The drawing under review shows one solid part. Ordinate dimensions are in mm from its lowest x, y, z. Round coordinates to 2 decimals unless told otherwise and drop trailing zeros. Order: outer loops, then holes, each group sorted by start corner. A loop starts at its lowest first (then second) coordinate and runs counter-clockwise, first axis right, second up. Notation, with made-up numbers: M -18.75,32.5 L 28.25,32.5 A19 ccw 28.25,41.5 Z; hole C 22.25,85.5 d4. An arc over 180 degrees is marked long. Answer as a JSON object with one key per item and string values.
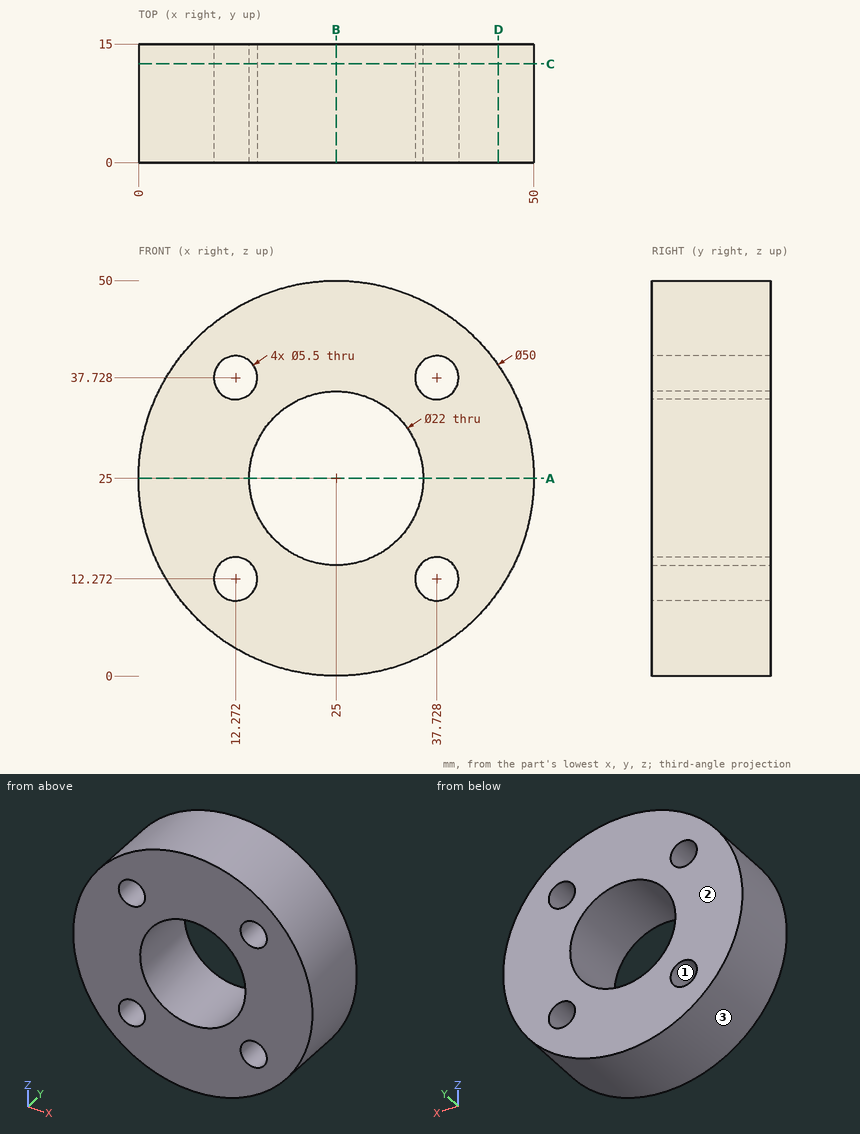
1) Add section D-D on x = 45.5. State the section outline as (y, z) points, and give its area (3 significant figures).
Geometry check:
{"outline": "M 0,10.69 L 15,10.69 L 15,39.31 L 0,39.31 Z", "area": "429 mm²"}
2) Insertion check: P1, Ø7, axis at x = 37.73, z = 12.27, coming from the -Y side; P2, Ø5, axis at x = 43.5, y = 12, coming from the -Z side; P3, Ø8, axis at x = 16.5, y = 13, coming from the -Z side; P4, Ø1, axis at x = 31, y = 12, coming from the +Z side. Each pin has a flat end and moves straight along its axis. Give the tip position at first contact, or say it passes through.
Geometry check:
{"P1": "stops at y = 0", "P2": "stops at z = 5.79", "P3": "stops at z = 0.41", "P4": "stops at z = 49.39"}
3) Add section A-A on z = 25. State the section outline as (x, y) points.
Geometry check:
{"outline": "M 0,0 L 14,0 L 14,15 L 0,15 Z; M 36,0 L 50,0 L 50,15 L 36,15 Z"}
4) Mouldability with a two-part tool opening along X and no side actions: class the marked faces 1, 2 and 3 as +X half, -X half, draft (parallel to the pull), parting line (faces both ways), or undercut.
Geometry check:
{"face 1": "undercut", "face 2": "draft", "face 3": "parting line"}
5) Add section C-C on y = 12.5. State the section outline as (x, z) points, and give its area (3 significant figures).
Geometry check:
{"outline": "C 25,25 d50; hole C 12.27,12.27 d5.5; hole C 12.27,37.73 d5.5; hole C 25,25 d22; hole C 37.73,12.27 d5.5; hole C 37.73,37.73 d5.5", "area": "1,490 mm²"}
6) For L1, parallel to Z at x = 24.5, y = 8.25 (1 decimal); L2, parallel to X at y = 8, z = 13, list the stretches that pass through material, from the lowest coordinate up.
Geometry check:
{"L1": "z = 0 to 14, 36 to 50", "L2": "x = 3.07 to 9.62, 14.92 to 35.08, 40.38 to 46.93"}
7) Add section B-B on x = 25. State the section outline as (y, z) points, and give its area (3 significant figures).
Geometry check:
{"outline": "M 0,0 L 15,0 L 15,14 L 0,14 Z; M 0,36 L 15,36 L 15,50 L 0,50 Z", "area": "420 mm²"}
